Check sheet for the modelled part. Datum: model origin and axes. Units: mm. Face numbers are marked on the shaded views. A direction names the side the tool comes from. Give positions to 0.01 mm unless a question says otherwise; leave off trailing zeros. Order: outer loops, then holes, each group sorted by start corner. A loop starts at its lowest first (then second) coordinate and runs counter-clockwise, first axis right, second up. Notation, with made-up numbers: (76, -32.5) -> (99, -32.5) arc R21 ccw to (99, -27.5) -> close; hole circle Ø11 at (-15.75, 24.25). An arc over 180 degrees is marked (long way). Answer in a Markdown table with one row per item. Add a question column.
(1) Cross-section at A-A (x = -76). Record the cut outline in (y, z).
(2) Cross-section at B-B (z = 142). Record the cut outline in (x, y).
(3) Set-up check for the marked faces 1 and 2: record each of +Z, -Z, +X, -X, +Y, -Y from which the full face is reachable in a straight line by a thin tool's end or side.
(4) Thickness scan on L1, parallel to X at y = -498.1, z = 100; L2, parallel to Y at x = -55.5, z = 68; L3, parallel to Z at x = -98, y = 14.5. Record the ranges inside material, lowest first. Write a range as [from, to].
(5) Cross-section at C-C (y = 230.5). Record the cut outline in (x, z), then the cut area to 3 significant figures.
(6) Go/stop test with flat-tipped pins: pin 1 (10 mm diameter, centred on x = -127, y = 276.5, fed in from +Z); pin 2 (9 mm diameter, centred on x = -100, z = 100, fed in from -Y). Record where each tip stops, or that it passes through.
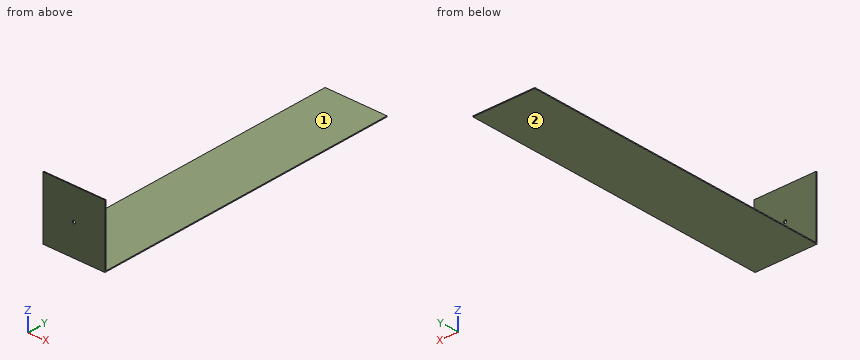
```python
from build123d import *

# Parameters (mm, degrees)
EXTRUDE_THIN1_DEPTH = 200
SKETCH2_R           = 5
CUT_EXTRUDE1_DEPTH  = 10


with BuildPart() as part:
    # Sketch1 → Extrude-Thin1 (new body)
    with BuildSketch(Plane(origin=(0, 0, 0), x_dir=(0, 0, -1), z_dir=(1, 0, 0))):
        Polygon((0, 500), (0, -500), (-200, -500), (-200, -497), (-3, -497), (-3, 500), align=None)
    extrude(amount=-EXTRUDE_THIN1_DEPTH)

    # Sketch2 → Cut-Extrude1 (cut)
    with BuildSketch(Plane.XZ.offset(500)):
        with Locations(Location((-100, 100, 0), (0, 0, 270))):
            Circle(SKETCH2_R)
    extrude(amount=-CUT_EXTRUDE1_DEPTH, mode=Mode.SUBTRACT)


solid = part.part
```
Answer below:
| question | item | result |
|---|---|---|
| 1 | outline | (-500, 0) -> (500, 0) -> (500, 3) -> (-497, 3) -> (-497, 200) -> (-500, 200) -> close |
| 2 | outline | (-200, -500) -> (0, -500) -> (0, -497) -> (-200, -497) -> close |
| 3 | face 1 | +Z, +X, -X, +Y |
| 3 | face 2 | -Z, +X, -X, +Y, -Y |
| 4 | L1 | x = [-200, -105], [-95, 0] |
| 4 | L2 | y = [-500, -497] |
| 4 | L3 | z = [0, 3] |
| 5 | outline | (-200, 0) -> (0, 0) -> (0, 3) -> (-200, 3) -> close |
| 5 | area | 600 mm² |
| 6 | pin 1 | stops at z = 3 |
| 6 | pin 2 | passes through |
